Geometry check sheet. Reference: drawing and pictorial views, mm from the part's lowest x, y, z. Round coordinates to 2 decimals unless told otherwise and drop trailing zeros. Write each loop counter-clockwise with the first axis right and the second up, starting at its lowest first coordinate (ties: lowest second). Pieces come first, ordered by that corner, then holes. Notation, with made-up numbers: M 42,48.25 L 74,48.25 A24 cw 74,70.25 Z; hole C 84,61.5 d2. An arc over 180 degrees is marked long. Answer in a Markdown table with one row per item. Add a question column.
1. Sectioned sample at C-C on y = 43.5. Record the cut outline in (x, z).
2. Sectioned sample at B-B on z = 50.8. Record the cut outline in (x, y), plus the area to 3 significant figures.
3. Material ranges on probe 1 along X at (y, z) = (15, 50.8); probe 2 along Y at (x, z) = (68, 46), recorded low to high.
4. Draft check along X on the marked faces 1, 2 and 3. Enter one of: pulls with the +X half, pulls with the -X half, needs draft (parallel to the pull), parting line crosses it, or undercut.
5. Go/stop test with flat-tipped pins: pin 1 Ø1 at (x, y) = (29.5, 48.5) entering from +Z; pin 2 Ø2 at (x, z) = (28, 41.5) entering from -Y; pin 3 Ø4 at (x, y) = (18, 27) entering from -Z. Record where each tip stops, or that it passes through.
6. Sectioned sample at A-A on x = 50.8. Record the cut outline in (y, z).
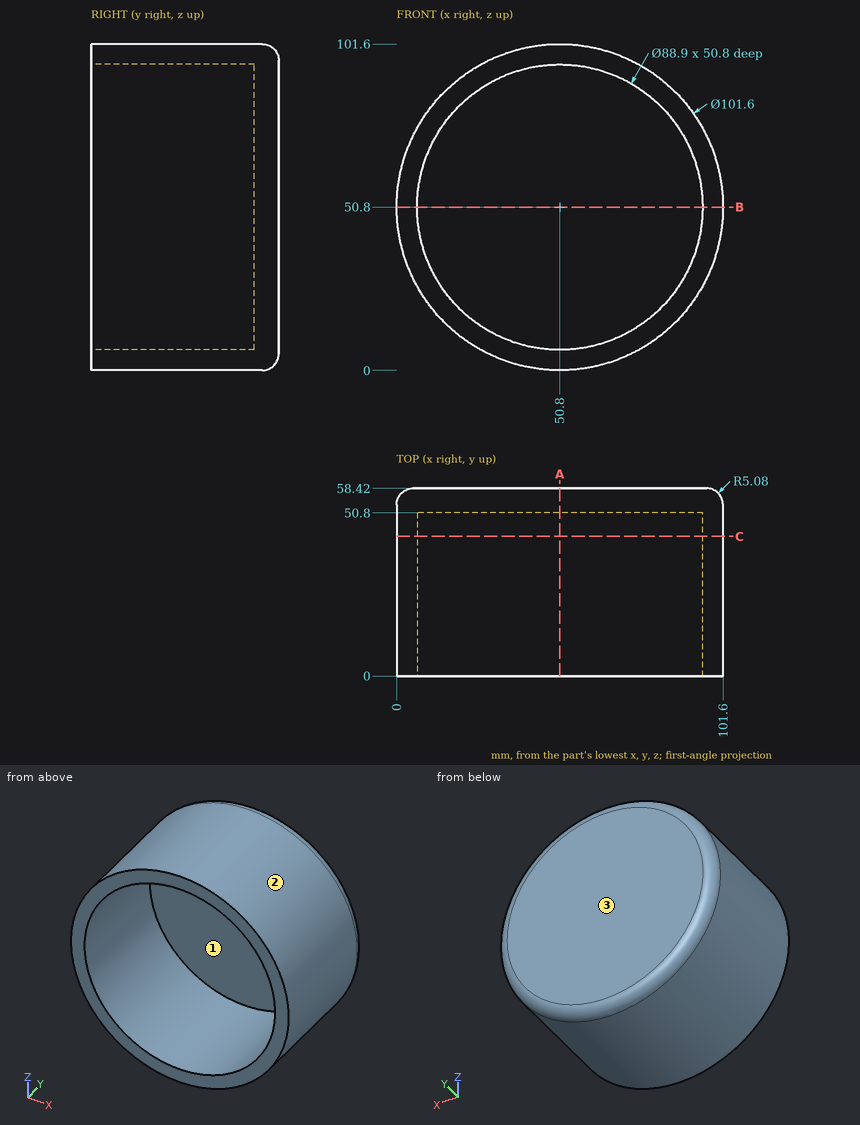
Geometry check:
| question | item | result |
|---|---|---|
| 1 | outline | C 50.8,50.8 d101.6; hole C 50.8,50.8 d88.9 |
| 2 | outline | M 0,0 L 6.35,0 L 6.35,50.8 L 95.25,50.8 L 95.25,0 L 101.6,0 L 101.6,53.34 A5.08 ccw 96.52,58.42 L 5.08,58.42 A5.08 ccw 0,53.34 Z |
| 2 | area | 1,410 mm2 |
| 3 | probe 1 | x = 0 to 6.35, 95.25 to 101.6 |
| 3 | probe 2 | y = 50.8 to 58.42 |
| 4 | face 1 | undercut |
| 4 | face 2 | parting line crosses it |
| 4 | face 3 | needs draft |
| 5 | pin 1 | stops at z = 97.15 |
| 5 | pin 2 | stops at y = 50.8 |
| 5 | pin 3 | stops at z = 10.4 |
| 6 | outline | M 0,0 L 53.34,0 A5.08 ccw 58.42,5.08 L 58.42,96.52 A5.08 ccw 53.34,101.6 L 0,101.6 L 0,95.25 L 50.8,95.25 L 50.8,6.35 L 0,6.35 Z |
